Check sheet for the modelled part. Datum: model origin and axes. Units: mm. A direction names the side the tool comes from. Round coordinates to 2 decimals unless told otherwise and drop trailing zeros. Write each loop counter-clockwise with the first axis right and the second up, starting at its lowest first coordinate (ties: lowest second). Pieces come first, ordered by that corner, then holes.
from build123d import *

# Parameters (mm, degrees)
ESQUISSE1_W         = 44
ESQUISSE1_H         = 15
BOSS_EXTRU_1_DEPTH  = 1.5
ESQUISSE2_W         = 6
ESQUISSE2_H         = 10
BOSS_EXTRU_2_DEPTH  = 2
CUT_EXTRUDE1_REACH  = 48.618
SKETCH1_R           = 1
SKETCH2_W           = 5.336665058
SKETCH2_H           = 9.146011637
BOSS_EXTRUDE1_DEPTH = 6


with BuildPart() as part:
    # Esquisse1 → Boss.-Extru.1 (new body)
    with BuildSketch(Plane.XY):
        with Locations((22, 7.5)):
            Rectangle(ESQUISSE1_W, ESQUISSE1_H)
    extrude(amount=BOSS_EXTRU_1_DEPTH)

    # Esquisse2 → Boss.-Extru.2 (add)
    with BuildSketch(Plane(origin=(0, 0, 0), x_dir=(-1, 0, 0), z_dir=(0, 0, -1))):
        with Locations((-41, 7.5)):
            Rectangle(ESQUISSE2_W, ESQUISSE2_H)
    extrude(amount=BOSS_EXTRU_2_DEPTH)

    # Sketch1 → Cut-Extrude1 (cut, up to next)
    with BuildSketch(Plane.XY.offset(1.5), mode=Mode.PRIVATE) as cut_extrude1_sk1:
        with Locations((44, 0)):
            Circle(SKETCH1_R)
    cut_extrude1_tool1 = extrude(cut_extrude1_sk1.sketch, amount=-CUT_EXTRUDE1_REACH, mode=Mode.PRIVATE) & part.part
    # Sketch1 → Cut-Extrude1 (cut, up to next)
    with BuildSketch(Plane.XY.offset(1.5), mode=Mode.PRIVATE) as cut_extrude1_sk2:
        with Locations((0, 15)):
            Circle(SKETCH1_R)
    cut_extrude1_tool2 = extrude(cut_extrude1_sk2.sketch, amount=-CUT_EXTRUDE1_REACH, mode=Mode.PRIVATE) & part.part
    add(cut_extrude1_tool1.solids().sort_by_distance((44, 0, 1.5))[0], mode=Mode.SUBTRACT)
    add(cut_extrude1_tool2.solids().sort_by_distance((0, 15, 1.5))[0], mode=Mode.SUBTRACT)

    # Sketch2 → Boss-Extrude1 (add)
    with BuildSketch(Plane(origin=(0, 0, 0), x_dir=(1, 0, 0), z_dir=(0, 0, -1))):
        with Locations((7.157544366, -7.402304661)):
            Rectangle(SKETCH2_W, SKETCH2_H)
    extrude(amount=BOSS_EXTRUDE1_DEPTH)


solid = part.part
1. Sectioned sample at C-C, the plane y = 7.5. Enter the section's corners in (x, z).
2. Release check for a two-part mould opening along X. For faces 1 (the flat face through (44, 8, 0)), 2 (the flat face through (9.826, 7, -3)), 3 (the flat face through (22, 8, 1.5)) record: released by +X, released by -X, zero draft, split by the parting line, or undercut.
3. Sectioned sample at D-D, the plane z = -4.25. Enter the section's corners in (x, y).
4. Scan lines: line 1 along X through (y, z) = (7, -1.25); line 2 along Z through (x, y) = (16, 9); line 3 along Y through (x, z) = (7.5, -2.5). Record each from-to range of solid material in increasing order.
5. Sectioned sample at A-A, the plane z = -0.5. Enter the section's corners in (x, y).
6. Sectioned sample at B-B, the plane x = 7. Enter the section's corners in (y, z).
7. Go/stop test with flat-tipped pins: pin 1 (3 mm diameter, centred on x = 41, y = 8, fed in from -Z); pin 2 (0.6 mm diameter, centred on x = 40.5, z = -1, fed in from +Y); pin 3 (0.6 mm diameter, centred on y = 9.5, z = -1.5, fed in from -X). Record where each tip stops, or that it passes through.
8. Set-up check for faces 4 (the flat face through (41, 12.5, -1)), 5 (the flat face through (7, 2.829, -3)), 6 (the flat face through (4.489, 7, -3)): record each of +Z, -Z, +X, -X, +Y, -Y from which the full face is reachable in a straight line by a thin tool's end or side.
Computed values:
1. outline: (0, 0) - (4.49, 0) - (4.49, -6) - (9.83, -6) - (9.83, 0) - (38, 0) - (38, -2) - (44, -2) - (44, 1.5) - (0, 1.5) - close
2. face 1: released by +X
2. face 2: undercut
2. face 3: zero draft
3. outline: (4.49, 2.83) - (9.83, 2.83) - (9.83, 11.98) - (4.49, 11.98) - close
4. line 1: x = 4.49 to 9.83, 38 to 44
4. line 2: z = 0 to 1.5
4. line 3: y = 2.83 to 11.98
5. outline: (4.49, 2.83) - (9.83, 2.83) - (9.83, 11.98) - (4.49, 11.98) - close; (38, 2.5) - (44, 2.5) - (44, 12.5) - (38, 12.5) - close
6. outline: (0, 0) - (2.83, 0) - (2.83, -6) - (11.98, -6) - (11.98, 0) - (15, 0) - (15, 1.5) - (0, 1.5) - close
7. pin 1: stops at z = -2
7. pin 2: stops at y = 12.5
7. pin 3: stops at x = 4.49
8. face 4: -Z, +X, -X, +Y
8. face 5: -Z, -X, -Y
8. face 6: -Z, -X, +Y, -Y
